Geometry check sheet. Reference: the model listing, model coordinates, mm. A direction names the side the tool comes from. Round coordinates to 2 decimals unless told otherwise and drop trailing zeros. Order: outer loops, then holes, each group sorted by start corner. A loop starts at its lowest first (then second) coordinate and runs counter-clockwise, first axis right, second up.
(1) Release check for a two-part mould opening along Z. For faces 1 (the face through (2.535, 20.633, 15.821)), 2 (the face through (20, 21, 0)), 3 (the face through (55, -19, -1)) record: +Z half, -Z half, draft (parallel to the pull), parting line (faces both ways), or undercut.
(2) Sectioned sample at A-A (x = 44). Record the boundary of the cut face in (y, z).
(3) Sectioned sample at B-B (z = 0). Give the number of separate pieces and of enclosed holes in the cut face, plus the area to 4 significant figures.
(4) Go/stop test with flat-tipped pins: pin 1 (1.5 mm diameter, centred on x = 35.5, z = 10, fed in from -Y); pin 2 (4.5 mm diameter, centred on x = 20, y = 0, fed in from -Z); pin 3 (4 mm diameter, centred on x = 19, y = 0.5, fed in from +Z). Record where each tip stops, or that it passes through.
(5) Material ranges on line 1 along X through (y, z) = (-20, -13); line 2 along X through (y, z) = (25, 19.5); line 3 along Z through (x, y) = (20, 23.7), recorded low to high.
(6) Set-up check for faces 4 (the face through (37.535, 20.633, 15.821)), 5 (the face through (7.54, -20.03, -6.31)), 6 (the face through (20, 0, 21)), 7 (the face through (17.5, -0.1, -23.5)), 8 (the face through (22.5, -23.5, -0.1)): record each of +Z, -Z, +X, -X, +Y, -Y from which the full face is reachable in a straight line by a thin tool's end or side.
(7) Sectioned sample at C-C (z = 12.5). Record the boundary of the cut face in (x, y).
from build123d import *

# Parameters (mm, degrees)
SKETCH2_R          = 17.5
CUT_EXTRUDE1_DEPTH = 85.113019206
SKETCH3_R          = 5
CUT_EXTRUDE2_DEPTH = 85.113019206
SKETCH4_R          = 2.5
CUT_EXTRUDE3_DEPTH = 5
SKETCH5_R          = 2.5
CUT_EXTRUDE4_DEPTH = 5
CUT_EXTRUDE5_START = -5
SKETCH6_R          = 2.5
CUT_EXTRUDE5_DEPTH = 5
CUT_EXTRUDE6_START = -5
SKETCH8_R          = 2.5
CUT_EXTRUDE6_DEPTH = 5


with BuildPart() as part:
    # Sketch1 → Revolve1 (revolve)
    with BuildSketch(Plane.XY, mode=Mode.PRIVATE) as revolve1_sk:
        Polygon((0, 0), (0, 26), (5, 26), (5, 21), (10, 21), (10, 26), (30, 26), (30, 21), (35, 21), (35, 26), (40, 26), (40, 45), (55, 45), (55, 0), align=None)
    revolve(revolve1_sk.sketch.rotate(Axis((0, 0, 0), (1, 0, 0)), 180), axis=Axis((0, 0, 0), (1, 0, 0)))

    # Sketch2 → Cut-Extrude1 (cut, through all)
    with BuildSketch(Plane.ZY):
        with Locations(Location((0, 0, 0), (0, 0, 270))):
            Circle(SKETCH2_R)
    extrude(amount=-CUT_EXTRUDE1_DEPTH, mode=Mode.SUBTRACT)

    # Sketch3 → Cut-Extrude2 (cut, through all)
    with BuildSketch(Plane(origin=(55, 0, 0), x_dir=(0, 0, -1), z_dir=(1, 0, 0))):
        with Locations(Location((-35, 0, 0), (0, 0, 90))):
            Circle(SKETCH3_R)
        with Locations(Location((0, 35, 0), (0, 0, 90))):
            Circle(SKETCH3_R)
        with Locations(Location((35, 0, 0), (0, 0, 90))):
            Circle(SKETCH3_R)
        with Locations(Location((0, -35, 0), (0, 0, 90))):
            Circle(SKETCH3_R)
    extrude(amount=-CUT_EXTRUDE2_DEPTH, mode=Mode.SUBTRACT)

    # Sketch4 → Cut-Extrude3 (cut)
    with BuildSketch(Plane(origin=(0, 26, 0), x_dir=(1, 0, 0), z_dir=(0, 1, 0))):
        with Locations(Location((20, 0, 0), (0, 0, 180))):
            Circle(SKETCH4_R)
    extrude(amount=-CUT_EXTRUDE3_DEPTH, mode=Mode.SUBTRACT)

    # Sketch5 → Cut-Extrude4 (cut)
    with BuildSketch(Plane.XY.offset(26)):
        with Locations((20, 0)):
            Circle(SKETCH5_R)
    extrude(amount=-CUT_EXTRUDE4_DEPTH, mode=Mode.SUBTRACT)

    # Sketch6 → Cut-Extrude5 (cut)
    with BuildSketch(Plane(origin=(0, -26, 0), x_dir=(-1, 0, 0), z_dir=(0, -1, 0)).offset(CUT_EXTRUDE5_START)):
        with Locations((-20, 0)):
            Circle(SKETCH6_R)
    extrude(amount=CUT_EXTRUDE5_DEPTH, mode=Mode.SUBTRACT)

    # Sketch8 → Cut-Extrude6 (cut)
    with BuildSketch(Plane(origin=(0, 0, -26), x_dir=(-1, 0, 0), z_dir=(0, 0, -1)).offset(CUT_EXTRUDE6_START)):
        with Locations(Location((-20, 0, 0), (0, 0, 180))):
            Circle(SKETCH8_R)
    extrude(amount=CUT_EXTRUDE6_DEPTH, mode=Mode.SUBTRACT)


solid = part.part
Answer below:
1. face 1: parting line
1. face 2: undercut
1. face 3: draft
2. outline: circle Ø90 at (0, 0); hole circle Ø10 at (-35, 0); hole circle Ø35 at (0, 0); hole circle Ø10 at (0, -35); hole circle Ø10 at (0, 35); hole circle Ø10 at (35, 0)
3. separate pieces: 4
3. enclosed holes: 0
3. area: 1,055 mm2
4. pin 1: stops at y = -24.3
4. pin 2: stops at z = -21
4. pin 3: stops at z = 26
5. line 1: x = 0 to 5, 10 to 30, 35 to 55
5. line 2: x = 40 to 55
5. line 3: z = -10.69 to -2.5, 2.5 to 10.69
6. face 4: -X
6. face 5: none
6. face 6: +Z
6. face 7: -Z
6. face 8: -Y
7. outline: (0, -22.8) - (5, -22.8) - (5, -16.87) - (10, -16.87) - (10, -22.8) - (30, -22.8) - (30, -16.87) - (35, -16.87) - (35, -22.8) - (40, -22.8) - (40, -43.23) - (55, -43.23) - (55, -12.25) - (0, -12.25) - close; (0, 12.25) - (55, 12.25) - (55, 43.23) - (40, 43.23) - (40, 22.8) - (35, 22.8) - (35, 16.87) - (30, 16.87) - (30, 22.8) - (10, 22.8) - (10, 16.87) - (5, 16.87) - (5, 22.8) - (0, 22.8) - close
